```python
from build123d import *

# Parameters (mm, degrees)
BOSS_EXTRUDE1_DEPTH = 2
M8_TAPPED_HOLE1_D   = 6.8
CUT_EXTRUDE1_DEPTH  = 2


with BuildPart() as part:
    # Sketch1 → Boss-Extrude1 (new body)
    with BuildSketch(Plane(origin=(0, 0, 0), x_dir=(1, 0, 0), z_dir=(0, 1, 0))):
        with BuildLine():
            Line((-57.325301205, 26.903614458), (142.674698795, 26.903614458))
            ThreePointArc((142.674698795, 26.903614458), (149.745766607, 23.97468227), (152.674698795, 16.903614458))
            Line((152.674698795, 16.903614458), (152.674698795, -88.096385542))
            ThreePointArc((152.674698795, -88.096385542), (149.745766607, -95.167453354), (142.674698795, -98.096385542))
            Line((142.674698795, -98.096385542), (-57.325301205, -98.096385542))
            ThreePointArc((-57.325301205, -98.096385542), (-64.396369017, -95.167453354), (-67.325301205, -88.096385542))
            Line((-67.325301205, -88.096385542), (-67.325301205, 16.903614458))
            ThreePointArc((-67.325301205, 16.903614458), (-64.396369017, 23.97468227), (-57.325301205, 26.903614458))
        make_face()
    extrude(amount=BOSS_EXTRUDE1_DEPTH)

    # M8 Tapped Hole1 (through all)
    with Locations(Plane(origin=(0, 2, 0), x_dir=(1, 0, 0), z_dir=(0, 1, 0))):
        with Locations((-57.325301205, 16.903614458), (142.674698795, 16.903614458), (-57.325301205, -88.096385542), (142.674698795, -88.096385542), (42.674698795, -88.096385542), (42.674698795, 16.903614458), (142.674698795, -35.596385542), (-57.325301205, -35.596385542)):
            Hole(M8_TAPPED_HOLE1_D / 2)

    # Sketch4 → Cut-Extrude1 (cut)
    with BuildSketch(Plane(origin=(0, 2, 0), x_dir=(1, 0, 0), z_dir=(0, 1, 0))):
        with BuildLine():
            Line((122.674698795, 6.903614458), (-37.325301205, 6.903614458))
            ThreePointArc((-37.325301205, 6.903614458), (-44.396369017, 3.97468227), (-47.325301205, -3.096385542))
            Line((-47.325301205, -3.096385542), (-47.325301205, -35.596385542))
            Line((-47.325301205, -35.596385542), (-47.325301205, -68.096385542))
            ThreePointArc((-47.325301205, -68.096385542), (-44.396369017, -75.167453354), (-37.325301205, -78.096385542))
            Line((-37.325301205, -78.096385542), (122.674698795, -78.096385542))
            ThreePointArc((122.674698795, -78.096385542), (129.745766607, -75.167453354), (132.674698795, -68.096385542))
            Line((132.674698795, -68.096385542), (132.674698795, -3.096385542))
            ThreePointArc((132.674698795, -3.096385542), (129.745766607, 3.97468227), (122.674698795, 6.903614458))
        make_face()
    extrude(amount=-CUT_EXTRUDE1_DEPTH, mode=Mode.SUBTRACT)


solid = part.part
```
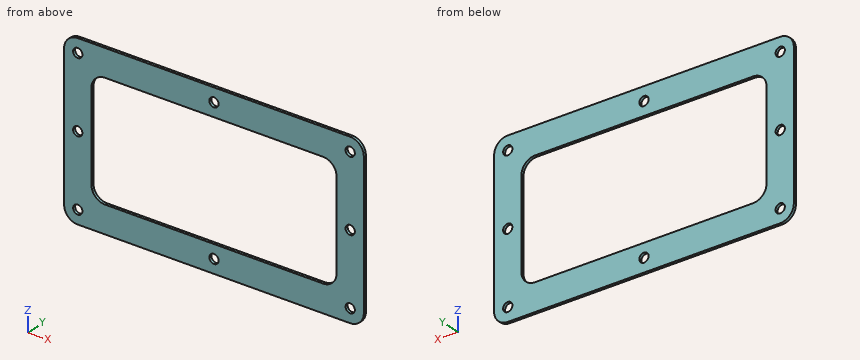
Model file for the job. Use its own axes, mm. Give positions to 0.01 mm unless a question says otherwise; leave off trailing zeros. Write each loop counter-clockwise with the first axis right and the second up, starting at its lowest first coordinate (ties: lowest second). Pieces come first, ordered by that corner, then holes. Notation, with made-up numbers: (1, 0) - (24, 0) arc R16 cw to (24, 5) - close; hole circle Ø8 at (-30.75, 45). An arc over 180 degrees is marked (long way). One line per question, with ' | ' between items. Start each with the question number.
(1) Wall check: line 1 along Z through (x, y) = (-57.5, 0.75); line 2 along Z through (x, y) = (7, 1.3); line 3 along X through (y, z) = (0.65, 31). Give the ranges that are in metal, low to high. Write a range as from..to.
(2) Slice it at A-A on x = 98.5. Write the cut outline in (y, z).
(3) Slice it at C-C on y = 1.05. Give the number of separate pieces and of enclosed holes in the cut face, plus the area to 3 significant figures.
(4) Pin check, flat tip, straight feed: P1, Ø6, axis at x = -57.33, z = -16.9, coming from the -Y side. Stop position of the tip, or through.
(5) Slice it at B-B on z = 42.5. Write the cut outline in (x, y).
Results below:
1) line 1: -26.9..-20.3, -13.51..32.2, 38.99..84.7, 91.49..98.09 | line 2: -26.9..-6.9, 78.1..98.1 | line 3: -67.33..-47.33, 132.67..152.67
2) outline: (0, -26.9) - (2, -26.9) - (2, -6.9) - (0, -6.9) - close; (0, 78.1) - (2, 78.1) - (2, 98.1) - (0, 98.1) - close
3) separate pieces: 1 | enclosed holes: 9 | area: 11,900 mm^2
4) P1: through
5) outline: (-67.33, 0) - (-47.33, 0) - (-47.33, 2) - (-67.33, 2) - close; (132.67, 0) - (152.67, 0) - (152.67, 2) - (132.67, 2) - close
